```python
from build123d import *

# Parameters (mm, degrees)
F1_DEPTH  = 406.4
F2_DEPTH  = 406.4
F0_W      = 812.8
F0_H      = 457.2
F3_DEPTH  = 228.6
F4_DEPTH  = 228.6
F5_R      = 203.2
F6_DEPTH  = 1270
F8_DEPTH  = 1270
F10_DEPTH = 812.8


with BuildPart() as f1:
    # F0 (on Top) → F1 (new body)
    with BuildSketch(Plane.XY):
        Polygon((1320.8, 0), (0, 0), (0, -279.4), (1041.4, -279.4), (1041.4, -736.6), (0, -736.6), (0, -1016), (1320.8, -1016), (1320.8, -736.6), (1320.8, -279.4), align=None)
    extrude(amount=F1_DEPTH)

    # F0 (on Top) → F2 (join)
    with BuildSketch(Plane.XY):
        Polygon((1320.8, 0), (0, 0), (0, -279.4), (1041.4, -279.4), (1041.4, -736.6), (0, -736.6), (0, -1016), (1320.8, -1016), (1320.8, -736.6), (1320.8, -279.4), align=None)
    extrude(amount=-F2_DEPTH)

    # F0 (on Top) → F3 (join)
    with BuildSketch(Plane.XY):
        with Locations((1727.2, -508)):
            Rectangle(F0_W, F0_H)
    extrude(amount=F3_DEPTH)

    # F0 (on Top) → F4 (join)
    with BuildSketch(Plane.XY):
        with Locations((1727.2, -508)):
            Rectangle(F0_W, F0_H)
    extrude(amount=-F4_DEPTH)

    # F5 (on face) → F6 (cut)
    with BuildSketch(Plane.XZ.offset(1016)):
        with Locations((406.4, 0)):
            Circle(F5_R)
    extrude(amount=-F6_DEPTH, mode=Mode.SUBTRACT)

    # F7 (on face) → F8 (cut)
    with BuildSketch(Plane.XZ.offset(1016)):
        with BuildLine():
            ThreePointArc((0, -2.103e-07), (119.0318040514, 287.3681957999), (406.4, 406.4))
            Line((406.4, 406.4), (0, 406.4))
            Line((0, 406.4), (0, -2.103e-07))
        make_face()
        with BuildLine():
            Line((0, -406.4), (406.4, -406.4))
            ThreePointArc((406.4, -406.4), (119.0318042001, -287.3681959486), (0, -2.103e-07))
            Line((0, -2.103e-07), (0, -406.4))
        make_face()
    extrude(amount=-F8_DEPTH, mode=Mode.SUBTRACT)

    # F9 (on face) → F10 (cut)
    with BuildSketch(Plane.YZ.offset(2133.6)):
        with BuildLine():
            ThreePointArc((-736.6, -8.745e-07), (-669.6446104884, 161.6446098701), (-508, 228.6))
            Line((-508, 228.6), (-736.6, 228.6))
            Line((-736.6, 228.6), (-736.6, -8.745e-07))
        make_face()
        with BuildLine():
            ThreePointArc((-508, 228.6), (-346.3553898208, 161.6446101792), (-279.4, 0))
            Line((-279.4, 0), (-279.4, 228.6))
            Line((-279.4, 228.6), (-508, 228.6))
        make_face()
        with BuildLine():
            Line((-279.4, -228.6), (-279.4, 0))
            ThreePointArc((-279.4, 0), (-346.3553898208, -161.6446101792), (-508, -228.6))
            Line((-508, -228.6), (-279.4, -228.6))
        make_face()
        with BuildLine():
            Line((-736.6, -228.6), (-508, -228.6))
            ThreePointArc((-508, -228.6), (-669.6446098701, -161.6446104884), (-736.6, -8.745e-07))
            Line((-736.6, -8.745e-07), (-736.6, -228.6))
        make_face()
    extrude(amount=-F10_DEPTH, mode=Mode.SUBTRACT)


solid = f1.part
```
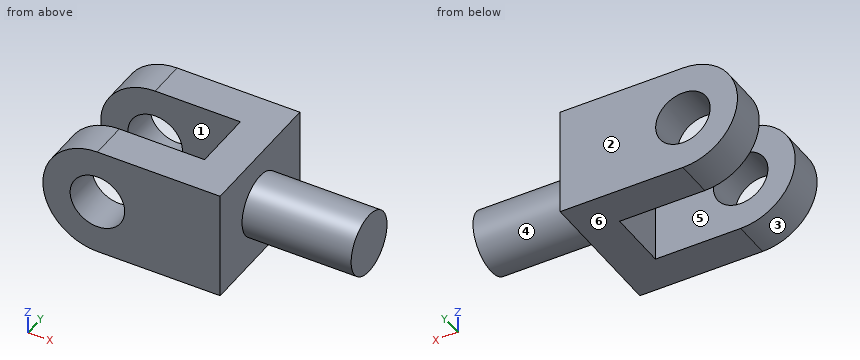
Build history of the part. All positions in model axes, mm. Face numbers are marked on the shaded views. A direction names the side the tool comes from. Round coordinates to 2 decimals unless told otherwise and drop trailing zeros. Loops run counter-clockwise (first coordinate to the right, second up) from the corner with the lowest first, then second, coordinate; pieces in that order, holes last.
Item 1: Saw through at B-B (y = -89.5). List the corners of the cut face in (x, z).
Item 2: Saw through at D-D (x = 275). List the corners of the cut face in (y, z), then the cut area to 3 significant figures.
Item 3: Drill centre lines: line 1 along Y through (x, z) = (691.5, 6); line 2 along Z through (x, y) = (406, -55); line 3 along X through (y, z) = (-319, -199.5). Where is each one in solid material? Low to high.
Item 4: Saw through at A-A (z = 0). List the corners of the cut face in (x, y).
Item 5: Two-plate mould, pull along Y, no slides. Class the marked faces 1, 2 and 3: released by +Y, released by -Y, zero draft, split by the parting line, or undercut.
Item 6: Which spindle directions (+Z, -Z, +X, -X, +Y, -Y) get a long thin tool onto all of the face, cutting with end or side? Do the marked faces 4, 5 and 6. Say none if no direction does.
Item 7: Saw through at C-C (x = 765). List the corners of the cut face in (y, z).
Item 8: Pin check, flat tip, straight feed: P1, Ø12, axis at y = -178, z = 297, coming from the +X side. Stop position of the tip, or through.
Worked answers:
1. outline: (406.4, -406.4) - (1320.8, -406.4) - (1320.8, 406.4) - (406.4, 406.4) arc R406.4 ccw to start; hole circle Ø406.4 at (406.4, 0)
2. outline: (-1016, -384.57) - (-736.6, -384.57) - (-736.6, -155) - (-1016, -155) - close; (-1016, 155) - (-736.6, 155) - (-736.6, 384.57) - (-1016, 384.57) - close; (-279.4, -384.57) - (0, -384.57) - (0, -155) - (-279.4, -155) - close; (-279.4, 155) - (0, 155) - (0, 384.57) - (-279.4, 384.57) - close
2. area: 257,000 mm2
3. line 1: y = -1016 to -736.6, -279.4 to 0
3. line 2: z = -406.4 to -203.2, 203.2 to 406.4
3. line 3: x = 1041.4 to 1320.8
4. outline: (0, -1016) - (203.2, -1016) - (203.2, -736.6) - (0, -736.6) - close; (0, -279.4) - (203.2, -279.4) - (203.2, 0) - (0, 0) - close; (609.6, -1016) - (1320.8, -1016) - (1320.8, -736.6) - (2133.6, -736.6) - (2133.6, -279.4) - (1320.8, -279.4) - (1320.8, 0) - (609.6, 0) - (609.6, -279.4) - (1041.4, -279.4) - (1041.4, -736.6) - (609.6, -736.6) - close
5. face 1: undercut
5. face 2: released by +Y
5. face 3: zero draft
6. face 4: +X
6. face 5: +Z, -Z, -X
6. face 6: -Z, +X, -X, +Y, -Y
7. outline: (-1016, -406.4) - (-736.6, -406.4) - (-736.6, 406.4) - (-1016, 406.4) - close; (-279.4, -406.4) - (0, -406.4) - (0, 406.4) - (-279.4, 406.4) - close
8. P1: stops at x = 1320.8
